Autodesk Fusion 360 part; units mm, degrees
sketch "Sketch1" plane through (0, 0, 0) normal (0, 1, 0) x (1, 0, 0)
  circle A0 centre (0, 0) radius 13.5
  circle A1 centre (0, 0) radius 19.35
  circle A2 centre (0, 0) radius 19.5
  circle A3 centre (0, 0) radius 23.3
  circle A4 centre (0, 0) radius 71
  line L0 (0, 0) -> (0, 71)
  line L1 (0, 0) -> (0, -71)
  line L2 (0, 0) -> (0.77, 0)
  line L3 (0.77, 0) -> (0.77, -76)
  line L4 (0.77, -76) -> (0, -76)
  line L5 (0, -76) -> (0, 0)
  line L6 (0, 0) -> (-0.77, 0)
  line L7 (-0.77, 0) -> (-0.77, -76)
  line L8 (-0.77, -76) -> (0, -76)
  line L9 (0, -76) -> (0, 0)
  line L10 (-0.77, 0) -> (0, 0)
  line L11 (0, 0) -> (0, 73)
  line L12 (0, 73) -> (-0.77, 73)
  line L13 (-0.77, 73) -> (-0.77, 0)
  line L14 (0, 73) -> (0.77, 73)
  line L15 (0.77, 73) -> (0.77, 0)
  line L16 (0.77, 0) -> (0, 0)
  line L17 (0, 0) -> (0, 73)
  line L18 (0, 0) -> (0, 35)
  line L19 (0, 0) -> (0, -35)
  line L20 (-0.77, 35) -> (-2, 35)
  line L21 (-2, 35) -> (-2, 62)
  line L22 (-2, 62) -> (-0.77, 62)
  line L23 (-0.77, 62) -> (-0.77, 35)
  line L24 (0.77, 35) -> (2, 35)
  line L25 (2, 35) -> (2, 62)
  line L26 (2, 62) -> (0.77, 62)
  line L27 (0.77, 62) -> (0.77, 35)
  line L28 (0.77, -35.0032) -> (2, -35.0032)
  line L29 (2, -35.0032) -> (2, -62)
  line L30 (2, -62) -> (0.77, -62)
  line L31 (0.77, -62) -> (0.77, -35.0032)
  line L32 (-0.77, -34.7868) -> (-2, -34.7868)
  line L33 (-2, -34.7868) -> (-2, -62)
  line L34 (-2, -62) -> (-0.77, -62)
  line L35 (-0.77, -62) -> (-0.77, -34.7868)
  line L36 (0, 0) -> (65.1081, -28.3184)
  line L37 (0, 0) -> (-28.3184, -65.1081)
  line L38 (-28.3184, -65.1081) -> (28.3184, 65.1081)
  line L39 (28.3184, 65.1081) -> (24.3299, 55.938)
  line L40 (0, 0) -> (-65.1081, 28.3184)
  line L41 (-65.1081, 28.3184) -> (-55.938, 24.3299)
  line L42 (65.1081, -28.3184) -> (55.938, -24.3299)
  line L43 (-28.3184, -65.1081) -> (-24.3299, -55.938)
  line L44 (-55.938, 24.3299) -> (-53.9437, 28.9149)
  line L45 (24.3299, 55.938) -> (28.9149, 53.9437)
  line L46 (55.938, -24.3299) -> (57.9322, -19.7448)
  line L47 (-24.3299, -55.938) -> (-19.7448, -57.9322)
  line L48 (-53.9437, 28.9149) -> (-62.9522, 32.8331)
  line L49 (-53.9437, 28.9149) -> (-57.9322, 19.7448)
  line L50 (-57.9322, 19.7448) -> (-66.9407, 23.663)
  line L51 (-24.3299, -55.938) -> (-28.9149, -53.9437)
  line L52 (-28.9149, -53.9437) -> (-32.8331, -62.9522)
  line L53 (-19.7448, -57.9322) -> (-23.663, -66.9407)
  line L54 (57.9322, -19.7448) -> (66.9407, -23.663)
  line L55 (55.938, -24.3299) -> (53.9437, -28.9149)
  line L56 (53.9437, -28.9149) -> (62.9522, -32.8331)
  line L57 (28.9149, 53.9437) -> (32.8331, 62.9522)
  line L58 (24.3299, 55.938) -> (19.7448, 57.9322)
  line L59 (19.7448, 57.9322) -> (23.663, 66.9407)
  circle A5 centre (0, 0) radius 25
  dimension "d1" = 27
  dimension "d2" = 38.7
  dimension "d3" = 39
  dimension "d4" = 46.6
  dimension "d5" = 142
  dimension "d6" = 0.77
  dimension "d7" = 0.77
  dimension "d8" = 35
  dimension "d9" = 35
  dimension "d10" = 10
  dimension "d11" = 10
  dimension "d12" = 10
  dimension "d13" = 10
  dimension "d14" = 5
  dimension "d15" = 5
  dimension "d16" = 5
  dimension "d17" = 5
  dimension "d18" = 10
  dimension "d19" = 5
  dimension "d20" = 5
  dimension "d21" = 5
  dimension "d22" = 50
extrude "Extrude1" add sketch "Sketch1" along normal blind 3 contours A4 L15 L24 L25 L26 L38 L58 L59 A5 | A4 L36 L38 L45 L46 L54 L57 A5 | A4 L3 L28 L29 L30 L36 L55 L56 A5 | A4 L0 L11 L15 L17 L18 L27 A5 | A4 L38 L39 L58 L59 | A4 L38 L39 L45 L57 | A4 L1 L3 L5 L9 L19 L31 A5 | A4 L36 L42 L46 L54 | A4 L36 L42 L55 L56 | A4 L0 L11 L13 L17 L18 L23 A5 | L15 L24 L25 L26 L27 | A4 L1 L5 L7 L9 L19 L35 A5 | L3 L28 L29 L30 L31 | A4 L13 L20 L21 L22 L40 L44 L48 L49 A5 | A4 L7 L32 L33 L34 L37 L38 L47 L53 A5 | A4 L37 L38 L40 L49 L50 L51 L52 A5 | L13 L20 L21 L22 L23 | L7 L32 L33 L34 L35 | A4 L40 L41 L49 L50 | A4 L40 L41 L44 L48 L49 | A4 L37 L38 L43 L47 L53 | A4 L37 L38 L43 L51 L52
extrude "Extrude2" add sketch "Sketch1" along normal blind 13 contours A4 L38 L39 L58 L59 | A4 L38 L39 L45 L57 | A4 L36 L42 L46 L54 | A4 L36 L42 L55 L56 | A4 L40 L41 L49 L50 | A4 L40 L41 L44 L48 L49 | A4 L37 L38 L43 L47 L53 | A4 L37 L38 L43 L51 L52
extrude "Extrude3" add sketch "Sketch1" along normal blind 8 contours L15 L24 L25 L26 L27 | L3 L28 L29 L30 L31 | L13 L20 L21 L22 L23 | L7 L32 L33 L34 L35
extrude "Extrude4" add 1 faces at (37.708, 3, 34.8341) along direction (0, 1, 0) blind 1
sketch "Sketch2" plane through (0, 4, 0) normal (0, 1, 0) x (-1, 0, 0)
  line L0 (-0.77, -62) -> (-2, -62)
  line L1 (-2, -62) -> (-2, -35)
  line L2 (-2, -35) -> (-0.77, -35)
  line L3 (-0.77, -35) -> (-0.77, -62)
  line L4 (0.77, 62) -> (2, 62)
  line L5 (2, 62) -> (2, 34.7868)
  line L6 (2, 34.7868) -> (0.77, 34.7868)
  line L7 (0.77, 34.7868) -> (0.77, 62)
  line L8 (0.77, -62) -> (0.77, -35)
  line L9 (0.77, -35) -> (2, -35)
  line L10 (2, -35) -> (2, -62)
  line L11 (2, -62) -> (0.77, -62)
  line L12 (-0.77, 62) -> (-0.77, 35.0032)
  line L13 (-0.77, 35.0032) -> (-2, 35.0032)
  line L14 (-2, 35.0032) -> (-2, 62)
  line L15 (-2, 62) -> (-0.77, 62)
  circle A0 centre (0, 0) radius 25
  line L16 (-62.9522, 32.8331) -> (-53.9437, 28.9149)
  line L17 (-53.9437, 28.9149) -> (-57.9322, 19.7448)
  line L18 (-57.9322, 19.7448) -> (-66.9407, 23.663)
  arc A1 (-66.9407, 23.663) -> (-32.8331, -62.9522) centre (0, 0) ccw
  line L19 (-32.8331, -62.9522) -> (-28.9149, -53.9437)
  line L20 (-28.9149, -53.9437) -> (-19.7448, -57.9322)
  line L21 (-19.7448, -57.9322) -> (-23.663, -66.9407)
  arc A2 (-23.663, -66.9407) -> (62.9522, -32.8331) centre (0, 0) ccw
  line L22 (62.9522, -32.8331) -> (53.9437, -28.9149)
  line L23 (53.9437, -28.9149) -> (57.9322, -19.7448)
  line L24 (57.9322, -19.7448) -> (66.9407, -23.663)
  arc A3 (66.9407, -23.663) -> (32.8331, 62.9522) centre (0, 0) ccw
  line L25 (32.8331, 62.9522) -> (28.9149, 53.9437)
  line L26 (28.9149, 53.9437) -> (19.7448, 57.9322)
  line L27 (19.7448, 57.9322) -> (23.663, 66.9407)
  arc A4 (23.663, 66.9407) -> (-62.9522, 32.8331) centre (0, 0) ccw
  line L28 (0, 0) -> (-20, -40)
  circle A5 centre (-20, -40) radius 8
  line L29 (-20, -40) -> (-12.8446, -43.5777)
  line L30 (-20, -40) -> (-54.5328, -19.2256)
  line L31 (-26.8552, -35.8761) -> (-34.2244, -31.4428)
  line L32 (-34.2244, -31.4428) -> (-41.0796, -27.3189)
  circle A6 centre (-41.0796, -27.3189) radius 8
  dimension "d31" = 16
  dimension "d32" = 40.3
  dimension "d33" = 8.6
  dimension "d34" = 8
  dimension "d35" = 16
extrude "Extrude5" cut sketch "Sketch2" against normal blind 36 contours L30 L32 A6 | L30 L32 A6 | L28 A5 L29 | L28 A5 L30 | A5 L29 L30
extrude "Extrude6" add sketch "Sketch1" along normal blind 1 contours A0 A1 L36 L38 | A0 A1 L15 L38 | A0 A1 L3 L36 | A0 A1 L0 L11 L15 L17 L18 | A1 A2 L36 L38 | A1 A2 L15 L38 | A0 A1 L1 L3 L5 L9 L19 | A1 A2 L3 L36 | A0 A1 L0 L11 L13 L17 L18 | A1 A2 L0 L11 L15 L17 L18 | A2 A3 L36 L38 | A2 A3 L15 L38 | A0 A1 L1 L5 L7 L9 L19 | A1 A2 L1 L3 L5 L9 L19 | A2 A3 L3 L36 | A0 A1 L13 L40 | A1 A2 L0 L11 L13 L17 L18 | A2 A3 L0 L11 L15 L17 L18 | A3 L36 L38 A5 | A3 L15 L38 A5 | A0 A1 L7 L37 L38 | A1 A2 L1 L5 L7 L9 L19 | A2 A3 L1 L3 L5 L9 L19 | A3 L3 L36 A5 | A0 A1 L37 L38 L40 | A1 A2 L13 L40 | A2 A3 L0 L11 L13 L17 L18 | A3 L0 L11 L15 L17 L18 A5 | A1 A2 L7 L37 L38 | A2 A3 L1 L5 L7 L9 L19 | A3 L1 L3 L5 L9 L19 A5 | A1 A2 L37 L38 L40 | A2 A3 L13 L40 | A3 L0 L11 L13 L17 L18 A5 | A2 A3 L7 L37 L38 | A3 L1 L5 L7 L9 L19 A5 | A2 A3 L37 L38 L40 | A3 L13 L40 A5 | A3 L7 L37 L38 A5 | A3 L37 L38 L40 A5
sketch "Sketch3" plane through (0, 0, 0) normal (0, 0, 1) x (1, 0, 0)
  line L0 (4.4303, 3.3085) -> (13.6469, 3.3085)
  line L1 (13.6469, 3.3085) -> (13.6469, 1.0043)
  line L2 (13.6469, 1.0043) -> (4.4303, 1.0043)
  line L3 (4.4303, 1.0043) -> (4.4303, 3.3085)
extrude "Extrude7" cut sketch "Sketch3" against normal blind 35
sketch "Sketch4" plane through (0, 1, 0) normal (0, 1, 0) x (-1, 0, 0)
  circle A0 centre (0, 0) radius 25
  circle A1 centre (-5.7905, -31.8479) radius 4.9823
sketch "Sketch5" plane through (0, 1, 0) normal (0, 1, 0) x (-1, 0, 0)
sketch "Sketch6" plane through (0, 0, 0) normal (0, 0, 1) x (1, 0, 0)
  circle A0 centre (0, 8.5) radius 1.5
  dimension "d42" = 3
extrude "Extrude8" cut sketch "Sketch1" along normal blind 28 contours A0 L3 L15 L36 L38 | A0 L15 L38 | A0 L3 L36 | A0 L0 L11 L15 L17 L18 L38 | L2 L15 L16 L38 | A0 L1 L3 L5 L9 L19 L36 | L2 L3 L16 L36 | A0 L0 L11 L13 L17 L18 L40 | L6 L7 L10 L37 L38 | A0 L1 L5 L7 L9 L19 L37 L38 | L6 L10 L13 L40 | A0 L13 L40 | A0 L7 L13 L37 L38 L40 | A0 L7 L37 L38
extrude "Extrude9" add sketch "Sketch1" along normal blind 3 contours A2 A3 L3 L36 | A2 A3 L13 L40
Can you work these out from the model? Positions are in its coordinate system, mm. A direction names the side the tool comes from. Give positions to 0.01 mm unless a question says otherwise; leave off trailing zeros. Loops run counter-clockwise (first coordinate to the right, second up) from the corner with the lowest first, then second, coordinate; pieces in that order, holes last. Notation, with made-up numbers: (38.5, 54) -> (82.5, 54) arc R20 ccw to (82.5, 75) -> close; hole circle Ø6 at (47, 76). An arc over 180 degrees is marked (long way). Return JSON: item names as keys, results as strings.
Q1. I want a section at A-A, the plane z = 0. List the corners of the cut face in (x, y) for me.
Checks:
{"outline": "(-71, 0) -> (-13.5, 0) -> (-13.5, 1) -> (-25, 1) -> (-25, 4) -> (-71, 4) -> close; (13.5, 0) -> (71, 0) -> (71, 4) -> (25, 4) -> (25, 1) -> (13.5, 1) -> close"}
Q2. I want a section at B-B, the plane z = 42.5. List the corners of the cut face in (x, y) for me.
Checks:
{"outline": "(-56.87, 0) -> (56.87, 0) -> (56.87, 4) -> (2, 4) -> (2, 8) -> (0.77, 8) -> (0.77, 4) -> (-0.77, 4) -> (-0.77, 8) -> (-2, 8) -> (-2, 4) -> (-56.87, 4) -> close"}
Q3. I want a section at C-C, the plane x = -43. List the corners of the cut face in (y, z) for me.
Checks:
{"outline": "(0, -56.5) -> (4, -56.5) -> (4, 56.5) -> (0, 56.5) -> close"}
Q4. On a 3-axis mill with a long thin cutter (end or side, diameter ignored), from which of +Z, -Z, +X, -X, +Y, -Y can I reach the whole of each face in a straight line? I mean faces 4 (the face through (-11, 3, -17)), 5 (the face through (-58.385, 8.437, -30.847)), 6 (the face through (0.77, 6, 48)), 7 (the face through (58.385, 8.437, 30.847)). Say none if no direction works.
Checks:
{"face 4": "+Y", "face 5": "-Z, +X, +Y", "face 6": "+Z, -Z, +Y", "face 7": "+Z, -X, +Y"}
Q5. For pin 1 Ø1 at (x, z) = (1.5, 51.5) entering from +Y; pin 2 Ø4.5 at (y, z) = (5.5, 44.5) entering from -X; pin 3 Ø1.5 at (y, z) = (6.5, -51) entering from -X; pin 4 Ø4 at (x, y) = (46.5, 7) entering from +Z, each with a flat end and sliding along its axis, tell me the tip position at first contact or that it passes through.
Checks:
{"pin 1": "stops at y = 8", "pin 2": "stops at x = -56.63", "pin 3": "stops at x = -2", "pin 4": "passes through"}
Q6. We'd pull the mould along X, two halves only. Please class faces 1 (the face through (-21.676, 8.437, 62.373)), 2 (the face through (-2, 6, -48)), 3 (the face through (32.76, 3.52, -62.99)): released by +X, released by -X, zero draft, split by the parting line, or undercut.
Checks:
{"face 1": "undercut", "face 2": "released by -X", "face 3": "split by the parting line"}
Q7. I want a section at D-D, the plane z = -40. List the corners of the cut face in (x, y) for me.
Checks:
{"outline": "(-58.66, 0) -> (12, 0) -> (12, 4) -> (2, 4) -> (2, 8) -> (0.77, 8) -> (0.77, 4) -> (-0.77, 4) -> (-0.77, 8) -> (-2, 8) -> (-2, 4) -> (-58.66, 4) -> close; (28, 0) -> (58.66, 0) -> (58.66, 4) -> (28, 4) -> close"}
Q8. I need wall thicknesses on probe 1 along X at (y, z) = (0.4, 0); probe 2 along Z at (x, y) = (-20.5, 1.5); probe 3 along X at (y, z) = (7.5, 56). Which ranges of each line are inside material? Lowest first, please.
Checks:
{"probe 1": "x = -71 to -13.5, 13.5 to 71", "probe 2": "z = -67.98 to -14.31, -11.07 to -8.92, 14.31 to 67.98", "probe 3": "x = -29.81 to -24.19, -2 to -0.77, 0.77 to 2"}
